```python
from build123d import *

# Parameters (mm, degrees)
SKETCH_1_W      = 30
SKETCH_1_H      = 30
EXTRUDE_1_DEPTH = 3
SKETCH_2_W      = 3
SKETCH_2_H      = 30
EXTRUDE_2_DEPTH = 22
SKETCH_3_W      = 20
SKETCH_3_H      = 30
SKETCH_3_R      = 2
EXTRUDE_3_DEPTH = 3


with BuildPart() as part:
    # 草图1 → 凸台-拉伸1 (new body)
    with BuildSketch(Plane.XY):
        Rectangle(SKETCH_1_W, SKETCH_1_H)
    extrude(amount=EXTRUDE_1_DEPTH)

    # 草图2 → 凸台-拉伸2 (add)
    with BuildSketch(Plane.XY.offset(3)):
        with Locations((13.5, 0)):
            Rectangle(SKETCH_2_W, SKETCH_2_H)
    extrude(amount=EXTRUDE_2_DEPTH)

    # 草图3 → 凸台-拉伸3 (add)
    with BuildSketch(Plane.XY.offset(25)):
        with Locations((5, 0)):
            Rectangle(SKETCH_3_W, SKETCH_3_H)
        with Locations((0, 10)):
            Circle(SKETCH_3_R, mode=Mode.SUBTRACT)
        with Locations(Location((0, -10, 0), (0, 0, 180))):
            Circle(SKETCH_3_R, mode=Mode.SUBTRACT)
    extrude(amount=EXTRUDE_3_DEPTH)


solid = part.part
```
For this review, take the finished solid that the model builds, in its own axes (mm). A direction names the side the tool comes from. Coordinates: 2 decimals unless noted, no trailing zeros. Order: outer loops, then holes, each group sorted by start corner. A loop starts at its lowest first (then second) coordinate and runs counter-clockwise, first axis right, second up. Notation, with made-up numbers: (-23, 83) -> (8, 83) arc R34 ccw to (8, 114) -> close; hole circle Ø11 at (-2.75, 78.5). An arc over 180 degrees is marked (long way). Use CSV: the item, a comma, the result in double quotes. Start each with the question number.
Item 1: We need section A-A, the plane x = 0. Give the boundary of the cut face in (y, z), then the cut area to 3 significant figures.
Item 2: We need section D-D, the plane z = 10. Give the boundary of the cut face in (x, y), then the cut area to 3 significant figures.
Item 3: We need section C-C, the plane y = -6.75. Give the boundary of the cut face in (x, z), then the cut area to 3 significant figures.
Item 4: We need section B-B, the plane y = -10. Give the boundary of the cut face in (x, z).
Item 5: Wall thickness on probe 1 along Y at (x, z) = (0, 25.75); probe 2 along Z at (x, y) = (9.5, 10.75); probe 3 along X at (y, z) = (-10, 26): over which ranges is each line inside the solid? List them lowest first.
Item 6: Insertion check: pin 1 (3.5 mm diameter, centred on y = -6.5, z = 26, fed in from -X); pin 2 (1.5 mm diameter, centred on x = -11, y = -4.5, fed in from +Z). Each pin has a flat end and moves straight along its axis. Give the tip position at first contact, or say it passes through.
Item 7: For faces 1 (the face through (0, -12, 26)), 2 (the face through (-5, 0, 26)), 3 (the face through (-2, 0, 3)), 4 (the face through (-15, 0, 1)), 5 (the face through (0, 0, 0)), list the 3-axis set-ups (+Z, -Z, +X, -X, +Y, -Y) from which the entire face can be reached by the end or side of a thin tool; tool diameter is ignored.
Item 8: Draft analysis for pull direction X (two halves, no side actions). For faces 6 (the face through (12, 0, 14)), 7 (the face through (5, 0, 28)), 8 (the face through (0, 12, 26)), state which applies: pulls with the +X half, pulls with the -X half, needs draft (parallel to the pull), parting line crosses it, or undercut.
Derived:
1,outline,"(-15, 0) -> (15, 0) -> (15, 3) -> (-15, 3) -> close; (-15, 25) -> (-12, 25) -> (-12, 28) -> (-15, 28) -> close; (-8, 25) -> (8, 25) -> (8, 28) -> (-8, 28) -> close; (12, 25) -> (15, 25) -> (15, 28) -> (12, 28) -> close"
1,area,"156 mm^2"
2,outline,"(12, -15) -> (15, -15) -> (15, 15) -> (12, 15) -> close"
2,area,"90.0 mm^2"
3,outline,"(-15, 0) -> (15, 0) -> (15, 28) -> (-5, 28) -> (-5, 25) -> (12, 25) -> (12, 3) -> (-15, 3) -> close"
3,area,"216 mm^2"
4,outline,"(-15, 0) -> (15, 0) -> (15, 28) -> (2, 28) -> (2, 25) -> (12, 25) -> (12, 3) -> (-15, 3) -> close; (-5, 25) -> (-2, 25) -> (-2, 28) -> (-5, 28) -> close"
5,probe 1,"y = -15 to -12, -8 to 8, 12 to 15"
5,probe 2,"z = 0 to 3, 25 to 28"
5,probe 3,"x = -5 to -2, 2 to 15"
6,pin 1,"stops at x = -5"
6,pin 2,"stops at z = 3"
7,face 1,"+Z"
7,face 2,"+Z, -X, +Y, -Y"
7,face 3,"-X, +Y, -Y"
7,face 4,"+Z, -Z, -X, +Y, -Y"
7,face 5,"-Z, +X, -X, +Y, -Y"
8,face 6,"pulls with the -X half"
8,face 7,"needs draft"
8,face 8,"undercut"
